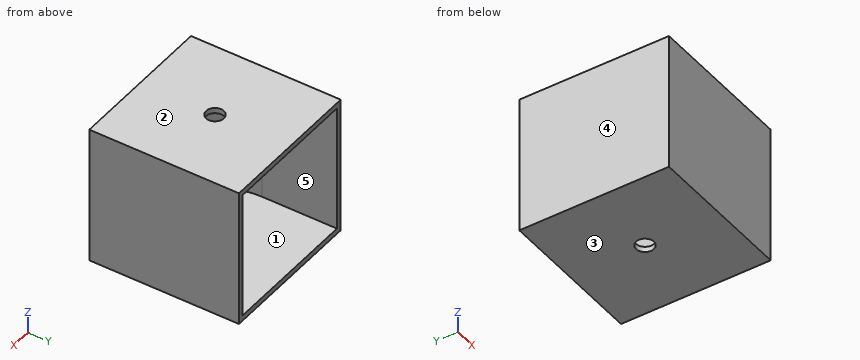
from build123d import *

# Parameters (mm, degrees)
SKETCH2_W           = 135
SKETCH2_H           = 135
SKETCH2_R           = 62.5
BOSS_EXTRUDE3_DEPTH = 5
SKETCH2_3_W         = 135
SKETCH2_3_H         = 135
BOSS_EXTRUDE4_DEPTH = 120
SKETCH3_W           = 125
SKETCH3_H           = 115
CUT_EXTRUDE1_DEPTH  = 67.5
SKETCH2_5_R         = 62.5
CUT_EXTRUDE2_DEPTH  = 115
CUT_EXTRUDE3_START  = 120
SKETCH2_6_R         = 8
CUT_EXTRUDE3_DEPTH  = 120


with BuildPart() as part:
    # Sketch2 → Boss-Extrude3 (new body)
    # profile 1 of 5: a face of its own
    with BuildSketch(Plane.XY):
        with Locations((67.5, 67.5)):
            Rectangle(SKETCH2_W, SKETCH2_H)
        with Locations((67.5, 67.5)):
            Circle(SKETCH2_R, mode=Mode.SUBTRACT)
    # profile 2 of 5: a face of its own
    with BuildSketch(Plane.XY):
        with BuildLine():
            Line((130, 67.5), (75.5, 67.5))
            ThreePointArc((75.5, 67.5), (67.5, 59.5), (59.5, 67.5))
            Line((59.5, 67.5), (5, 67.5))
            ThreePointArc((5, 67.5), (67.5, 5), (130, 67.5))
        make_face()
    # profile 3 of 5: a face of its own
    with BuildSketch(Plane.XY):
        with BuildLine():
            ThreePointArc((59.5, 67.5), (67.5, 75.5), (75.5, 67.5))
            Line((75.5, 67.5), (130, 67.5))
            ThreePointArc((130, 67.5), (67.5, 130), (5, 67.5))
            Line((5, 67.5), (59.5, 67.5))
        make_face()
    # profile 4 of 5: a face of its own
    with BuildSketch(Plane.XY):
        with BuildLine():
            Line((130, 67.5), (75.5, 67.5))
            ThreePointArc((75.5, 67.5), (67.5, 59.5), (59.5, 67.5))
            Line((59.5, 67.5), (5, 67.5))
            ThreePointArc((5, 67.5), (67.5, 5), (130, 67.5))
        make_face()
    # profile 5 of 5: a face of its own
    with BuildSketch(Plane.XY):
        with BuildLine():
            ThreePointArc((59.5, 67.5), (67.5, 75.5), (75.5, 67.5))
            Line((75.5, 67.5), (130, 67.5))
            ThreePointArc((130, 67.5), (67.5, 130), (5, 67.5))
            Line((5, 67.5), (59.5, 67.5))
        make_face()
    extrude(amount=-BOSS_EXTRUDE3_DEPTH)

    # Sketch2_3 → Boss-Extrude4 (add)
    with BuildSketch(Plane.XY):
        with Locations((67.5, 67.5)):
            Rectangle(SKETCH2_3_W, SKETCH2_3_H)
    extrude(amount=BOSS_EXTRUDE4_DEPTH)

    # Sketch3 → Cut-Extrude1 (cut)
    with BuildSketch(Plane(origin=(0, 135, 0), x_dir=(1, 0, 0), z_dir=(0, 1, 0))):
        with Locations((67.5, -57.5)):
            Rectangle(SKETCH3_W, SKETCH3_H)
    extrude(amount=-CUT_EXTRUDE1_DEPTH, mode=Mode.SUBTRACT)

    # Sketch2_5 → Cut-Extrude2 (cut)
    with BuildSketch(Plane.XY):
        with Locations((67.5, 67.5)):
            Circle(SKETCH2_5_R)
    extrude(amount=CUT_EXTRUDE2_DEPTH, mode=Mode.SUBTRACT)

    # Sketch2_6 → Cut-Extrude3 (cut)
    with BuildSketch(Plane.XY.offset(CUT_EXTRUDE3_START)):
        with Locations((67.5, 67.5)):
            Circle(SKETCH2_6_R)
    extrude(amount=-CUT_EXTRUDE3_DEPTH, mode=Mode.SUBTRACT)


solid = part.part
Can you work these out from the model? Positions are in its coordinate system, mm. Face numbers are marked on the shaded views. A direction names the side the tool comes from. Coordinates: 2 decimals unless noted, no trailing zeros. Loops run counter-clockwise (first coordinate to the right, second up) from the corner with the lowest first, then second, coordinate; pieces in that order, holes last. Notation, with made-up numbers: M 10.5,-35.5 L 27.5,-35.5 A18 cw 27.5,-6.5 Z; hole C 68,-20 d5. An arc over 180 degrees is marked long. Answer as CSV lines item,"result". Start each with the question number.
1. Thinking about a two-plate mould opening in Z: for the marked faces 3, 4 and 5, which applies, +Z half, -Z half, draft (parallel to the pull), parting line (faces both ways), or undercut?
2. For the marked faces 1 and 2, which set-ups out of +Z, -Z, +X, -X, +Y, -Y let a thin tool reach every point of the face, with its end or its side?
3. If I drill on probe 1 along Z at (x, y) = (81.5, 15.5); probe 2 along X at (y, z) = (86.5, 44); probe 3 along Y at (x, z) = (67.5, -1.6), over which ranges is the centre line in solid material (lowest first)? Write a range as [from, to].
4. Suppose I cut it at D-D, the plane x = 13. List the corners of the cut face in (y, z) for me.
5. Suppose I cut it at B-B, the plane x = 67.5. List the corners of the cut face in (y, z) for me.
6. For pin 1 Ø14.5 at (x, y) = (67.5, 67.5) entering from -Z; pin 2 Ø4 at (x, z) = (68.5, 98.5) entering from +Y, each with a flat end and sliding along its axis, tell me the tip position at first contact or that it passes through.
7. Suppose I cut it at C-C, the plane z = 42.5. List the corners of the cut face in (x, y) for me.
8. Suppose I cut it at A-A, the plane y = 30. List the corners of the cut face in (x, z) for me.
Output:
1,face 3,"-Z half"
1,face 4,"draft"
1,face 5,"undercut"
2,face 1,"+Y"
2,face 2,"+Z, +X, -X, +Y, -Y"
3,probe 1,"z = [-5, 0], [115, 120]"
3,probe 2,"x = [0, 5], [130, 135]"
3,probe 3,"y = [0, 59.5], [75.5, 135]"
4,outline,"M 0,-5 L 135,-5 L 135,0 L 36.91,0 L 36.91,115 L 135,115 L 135,120 L 0,120 Z"
5,outline,"M 0,-5 L 59.5,-5 L 59.5,0 L 5,0 L 5,115 L 59.5,115 L 59.5,120 L 0,120 Z; M 75.5,-5 L 135,-5 L 135,0 L 75.5,0 Z; M 75.5,115 L 135,115 L 135,120 L 75.5,120 Z"
6,pin 1,"passes through"
6,pin 2,"stops at y = 5.07"
7,outline,"M 0,0 L 135,0 L 135,135 L 130,135 L 130,67.5 A62.5 cw 5,67.5 L 5,135 L 0,135 Z"
8,outline,"M 0,-5 L 135,-5 L 135,120 L 0,120 Z; hole M 17.5,0 L 117.5,0 L 117.5,115 L 17.5,115 Z"
